CAD build for the part. Positions are in the model's coordinates, mm. A direction names the side the tool comes from. Coordinates: 2 decimals unless noted, no trailing zeros. Order: outer loops, then holes, each group sorted by start corner. A loop starts at its lowest first (then second) coordinate and runs counter-clockwise, first axis right, second up.
Autodesk Inventor part; units mm, degrees
ref_plane "YZ Plane" through (0, 0, 0) normal (1, 0, 0) x (0, 1, 0)
ref_plane "XZ Plane" through (0, 0, 0) normal (0, 1, 0) x (-1, 0, 0)
ref_plane "XY Plane" through (0, 0, 0) normal (0, 0, 1) x (1, 0, 0)
sketch "Sketch1" plane through (0, 0, 0) normal (0, 1, 0) x (-1, 0, 0)
  line L0 (0, 0) -> (76.2, 0)
  line L1 (76.2, 0) -> (76.2, -647.7)
  line L2 (76.2, -647.7) -> (0, -647.7)
  line L3 (0, -647.7) -> (0, 0)
  dimension "d1" = 76.2
  dimension "d2" = 647.7
extrude "Extrusion1" add sketch "Sketch1" along normal blind 19.05
sketch "Sketch2" plane through (0, 19.05, 0) normal (0, 1, 0) x (1, 0, 0)
  line L0 (-64.135, 554.99) -> (-12.065, 554.99)
  line L1 (-12.065, 554.99) -> (-12.065, 537.21)
  line L2 (-12.065, 537.21) -> (-64.135, 537.21)
  line L3 (-64.135, 537.21) -> (-64.135, 554.99)
  circle A0 centre (-64.135, 546.1) radius 8.89
  circle A1 centre (-12.065, 546.1) radius 8.89
  line L4 (-73.025, 606.1343) -> (-73.025, 587.8403) construction
  line L5 (-3.175, 554.99) -> (-3.175, 587.8403) construction
  line L6 (0, 647.7) -> (-76.2, 647.7)
  line L7 (-38.1, 647.7) -> (-38.1, 0) construction
  line L8 (-76.2, 0) -> (0, 0)
  dimension "d5" = 69.85
  dimension "d6" = 34.925
  dimension "d7" = 17.78
  dimension "d8" = 101.6
extrude "Extrusion2" cut sketch "Sketch2" against normal blind 25.4
sketch "Sketch3" plane through (0, 0, 0) normal (0, -1, 0) x (1, 0, 0)
  line L0 (0, 0) -> (0, -647.7)
  line L1 (-76.2, -647.7) -> (-76.2, 0)
  line L2 (0, -531.3622) -> (-76.2, -531.3622)
  line L3 (-76.2, -531.3622) -> (-76.2, -563.4771)
  line L4 (-76.2, -563.4771) -> (0, -563.4771)
  line L5 (0, -563.4771) -> (0, -531.3622)
  point P0 (0, -563.4771)
extrude "Extrusion3" cut sketch "Sketch3" against normal blind 12.7
equation "\"d1\" = topPlateWidth"
equation "\"d2\" = topPlateLength"
equation "\"d3\" = woodThickness"
equation "\"d6\" = 0.5 * d5"
equation "\"topPlateLength\" = 647.7"
equation "\"woodThickness\" = 19.05"
equation "\"topPlateWidth\" = 76.2"
properties part number "bodyTopPlate"
1) Drill centre lines: probe 1 along Z at (x, y) = (-46.5, 6.5); probe 2 along Z at (x, y) = (-13, 15). Where is each one in solid material? Low to high.
2) Two-plate mould, pull along Z, no slides. Class faces 1 (the flat face through (-76.2, 9, -319)), 2 (the flat face through (-39, 9, -647.7)), 3 (the flat face through (-39, 12.7, -558)): released by +Z, released by -Z, zero draft, split by the parting line, or undercut.
3) Slice it at B-B (z = -546.1). List the corners of the cut face in (x, y) (3 decimals), plus the area to 3 significant figures.
4) Slice it at C-C (x = -53.5). List the corners of the cut face in (y, z), plus the area to 3 significant figures.
5) Which spindle directions (+Z, -Z, +X, -X, +Y, -Y) get a long thin tool onto all of the face, cutting with end or side? Do faces 4 (the flat face through (-38, 6, -531.362)), 5 (the flat face through (-38, 0, -262)). Say none if no direction does.
6) Slice it at A-A (y = 8.5). List the corners of the cut face in (x, z).
Worked out:
1. probe 1: z = -647.7 to -563.48, -531.36 to 0
1. probe 2: z = -647.7 to -554.99, -537.21 to 0
2. face 1: zero draft
2. face 2: released by -Z
2. face 3: undercut
3. outline: (-76.2, 12.7) - (-73.025, 12.7) - (-73.025, 19.05) - (-76.2, 19.05) - close; (-3.175, 12.7) - (0, 12.7) - (0, 19.05) - (-3.175, 19.05) - close
3. area: 40.3 mm2
4. outline: (0, -647.7) - (19.05, -647.7) - (19.05, -554.99) - (12.7, -554.99) - (12.7, -563.48) - (0, -563.48) - close; (0, -531.36) - (12.7, -531.36) - (12.7, -537.21) - (19.05, -537.21) - (19.05, 0) - (0, 0) - close
4. area: 11,800 mm2
5. face 4: +X, -X, -Y
5. face 5: +Z, -Z, +X, -X, -Y
6. outline: (-76.2, -647.7) - (0, -647.7) - (0, -563.48) - (-76.2, -563.48) - close; (-76.2, -531.36) - (0, -531.36) - (0, 0) - (-76.2, 0) - close
